Geometry check sheet. Reference: the model listing, model coordinates, mm. A direction names the side the tool comes from. Coordinates: 2 decimals unless noted, no trailing zeros. Loops run counter-clockwise (first coordinate to the right, second up) from the corner with the lowest first, then second, coordinate; pieces in that order, holes last. Notation, with made-up numbers: (85.5, 4) -> (105.5, 4) arc R13 cw to (105.5, 13) -> close; hole circle Ø1 at (4, 75). An arc over 180 degrees is marked (long way). Answer as a JSON object with one key per item and string values.
from build123d import *

# Parameters (mm, degrees)
ESQUISSE1_R             = 20.5
BOSS_EXTRU_1_DEPTH      = 110
ESQUISSE2_OUTSIDE_W     = 67.87
ESQUISSE2_OUTSIDE_H     = 67.87
ESQUISSE2_OUTSIDE_R     = 18.95
ENL_V_MAT_EXTRU_1_DEPTH = 22
ESQUISSE3_OUTSIDE_W     = 67.87
ESQUISSE3_OUTSIDE_H     = 67.87
ESQUISSE3_OUTSIDE_R     = 19.95
ENL_V_MAT_EXTRU_2_DEPTH = 22
ESQUISSE5_R             = 5
ENL_V_MAT_EXTRU_3_DEPTH = 111
ESQUISSE6_R             = 2.5
ENL_V_MAT_EXTRU_4_DEPTH = 50
ESQUISSE7_R             = 2.5
ENL_V_MAT_EXTRU_5_DEPTH = 50


with BuildPart() as part:
    # Esquisse1 → Boss.-Extru.1 (new body)
    with BuildSketch(Plane(origin=(0, 0, 0), x_dir=(1, 0, 0), z_dir=(0, 1, 0))):
        Circle(ESQUISSE1_R)
    extrude(amount=BOSS_EXTRU_1_DEPTH)

    # Esquisse2 outside → Enlèv. mat.-Extru.1 (cut)
    with BuildSketch(Plane(origin=(0, 110, 0), x_dir=(1, 0, 0), z_dir=(0, 1, 0))):
        Rectangle(ESQUISSE2_OUTSIDE_W, ESQUISSE2_OUTSIDE_H)
        Circle(ESQUISSE2_OUTSIDE_R, mode=Mode.SUBTRACT)
    extrude(amount=-ENL_V_MAT_EXTRU_1_DEPTH, mode=Mode.SUBTRACT)

    # Esquisse3 outside → Enlèv. mat.-Extru.2 (cut)
    with BuildSketch(Plane.XZ):
        Rectangle(ESQUISSE3_OUTSIDE_W, ESQUISSE3_OUTSIDE_H)
        Circle(ESQUISSE3_OUTSIDE_R, mode=Mode.SUBTRACT)
    extrude(amount=-ENL_V_MAT_EXTRU_2_DEPTH, mode=Mode.SUBTRACT)

    # Esquisse5 → Enlèv. mat.-Extru.3 (cut, through all)
    with BuildSketch(Plane(origin=(0, 110, 0), x_dir=(1, 0, 0), z_dir=(0, 1, 0))):
        Circle(ESQUISSE5_R)
    extrude(amount=-ENL_V_MAT_EXTRU_3_DEPTH, mode=Mode.SUBTRACT)

    # Esquisse6 → Enlèv. mat.-Extru.4 (cut)
    with BuildSketch(Plane(origin=(0, 110, 0), x_dir=(1, 0, 0), z_dir=(0, 1, 0))):
        with Locations((0, -12.5)):
            Circle(ESQUISSE6_R)
        with Locations((-10.825317547, -6.25)):
            Circle(ESQUISSE6_R)
        with Locations((-10.825317547, 6.25)):
            Circle(ESQUISSE6_R)
        with Locations((0, 12.5)):
            Circle(ESQUISSE6_R)
        with Locations((10.825317547, 6.25)):
            Circle(ESQUISSE6_R)
        with Locations((10.825317547, -6.25)):
            Circle(ESQUISSE6_R)
    extrude(amount=-ENL_V_MAT_EXTRU_4_DEPTH, mode=Mode.SUBTRACT)

    # Esquisse7 → Enlèv. mat.-Extru.5 (cut)
    with BuildSketch(Plane.XZ):
        with Locations((10.825317547, -6.25)):
            Circle(ESQUISSE7_R)
        with Locations((0, -12.5)):
            Circle(ESQUISSE7_R)
        with Locations((-10.825317547, -6.25)):
            Circle(ESQUISSE7_R)
        with Locations((-10.825317547, 6.25)):
            Circle(ESQUISSE7_R)
        with Locations((0, 12.5)):
            Circle(ESQUISSE7_R)
        with Locations((10.825317547, 6.25)):
            Circle(ESQUISSE7_R)
    extrude(amount=-ENL_V_MAT_EXTRU_5_DEPTH, mode=Mode.SUBTRACT)


solid = part.part
1. Tool access check on faces 1 (the face through (-8.44, 24.65, -5.5)), 2 (the face through (4, 0, 4)), 3 (the face through (13.21, 85.35, -7)). Record the directions out of +Z, -Z, +X, -X, +Y, -Y that give a thin tool (end or side, any length) a straight path to the whole face; none if there is none.
Evaluation:
{"face 1": "-Y", "face 2": "+Z, -Z, +X, -X, -Y", "face 3": "+Y"}
2. Thickness scan on probe 1 along Z at (x, y) = (0, 25.5); probe 2 along Z at (x, y) = (12.5, 45); probe 3 along X at (y, z) = (66, -0.5). Record the ranges inside material, lowest first. Write a range as from..to.
Evaluation:
{"probe 1": "z = -20.5..-15, -10..-5, 5..10, 15..20.5", "probe 2": "z = -16.25..-8.11, -4.39..4.39, 8.11..16.25", "probe 3": "x = -20.49..-4.97, 4.97..20.49"}
3. Section check A-A, the plane y = 25. Record the boundary of the cut face in (x, z).
Evaluation:
{"outline": "circle Ø41 at (0, 0); hole circle Ø5 at (-10.83, -6.25); hole circle Ø5 at (-10.83, 6.25); hole circle Ø10 at (0, 0); hole circle Ø5 at (0, -12.5); hole circle Ø5 at (0, 12.5); hole circle Ø5 at (10.83, -6.25); hole circle Ø5 at (10.83, 6.25)"}
4. Section check D-D, the plane z = -6.25. Record the boundary of the cut face in (x, y).
Evaluation:
{"outline": "(-19.52, 22) -> (-18.95, 22) -> (-18.95, 0) -> (-13.33, 0) -> (-13.33, 50) -> (-8.33, 50) -> (-8.33, 0) -> (8.33, 0) -> (8.33, 50) -> (13.33, 50) -> (13.33, 0) -> (18.95, 0) -> (18.95, 22) -> (19.52, 22) -> (19.52, 88) -> (17.89, 88) -> (17.89, 110) -> (13.33, 110) -> (13.33, 60) -> (8.33, 60) -> (8.33, 110) -> (-8.33, 110) -> (-8.33, 60) -> (-13.33, 60) -> (-13.33, 110) -> (-17.89, 110) -> (-17.89, 88) -> (-19.52, 88) -> close"}
5. Section check C-C, the plane z = 0. Record the boundary of the cut face in (x, y), then the cut area to 3 significant figures.
Evaluation:
{"outline": "(-20.5, 22) -> (-19.95, 22) -> (-19.95, 0) -> (-5, 0) -> (-5, 110) -> (-18.95, 110) -> (-18.95, 88) -> (-20.5, 88) -> close; (5, 0) -> (19.95, 0) -> (19.95, 22) -> (20.5, 22) -> (20.5, 88) -> (18.95, 88) -> (18.95, 110) -> (5, 110) -> close", "area": "3,320 mm^2"}
6. Depth check by flat-ended pin: P1, Ø1.5, axis at x = -9.5, z = 6, coming from the +Y side; P2, Ø3, axis at x = 12, y = 67, coming from the -Z side; P3, Ø3, axis at x = 10.83, z = -6.25, coming from the -Y side. Enter the tip coordinate at first touch or a pass-through.
Evaluation:
{"P1": "stops at y = 60", "P2": "stops at z = -17.61", "P3": "stops at y = 50"}
7. Mould release check, pull along Z, two halves, no side actions. Record for faces 4 (the face through (14, 88, 14)), 5 (the face through (11, 50, 6)): released by +Z, released by -Z, zero draft, split by the parting line, or undercut.
Evaluation:
{"face 4": "zero draft", "face 5": "undercut"}
